Source: CAD feature listing. Evaluate the final solid. Frame: model axes, mm. A direction names the side the tool comes from. Round coordinates to 2 decimals unless told otherwise and drop trailing zeros. Loops run counter-clockwise (first coordinate to the right, second up) from the corner with the lowest first, then second, coordinate; pieces in that order, holes last.
Item 1: Section query B-B on z = 1.4. Return loops of the section in (x, y) (3 decimals), then the cut area to 3 significant figures.
Item 2: Section query D-D on y = 9. Return loops of the section in (x, z), then the cut area to 3 significant figures.
Item 3: Access query for faces 1 (the flat face through (40, 44, 3)), 2 (the flat face through (40, 5, 3)), 3 (the flat face through (-40, 44, 3)). Directions: +Z, -Z, +X, -X, +Y, -Y. A direction counts if a zero-diameter tool reaches every point of the face in a straight line with its end or side. Return the directions, or none.
Item 4: Section query C-C on x = -24. Return loops of the section in (y, z).
Item 5: Ray query, L1, parallel to Y at x = -21, z = 3.25; L2, parallel to X at y = 36, z = 3.6; L3, parallel to Y at x = -25, z = 5.3. Return the intervals inside material, ascending.
Item 6: Pull-direction query (X, two-part tool) for faces 4 (the flat face through (-40, 5, 3)), 5 (the cylindrical face through (22.21, 38.53, 2.96)), 6 (the flat face through (-43, 32, 3)); classes: released by +X, released by -X, zero draft, split by the parting line, or undercut.
Item 7: First-contact query: P1, Ø6.5, axis at x = 22.665, y = 42, coming from the -Z side; P2, Ø3, axis at y = 44, z = 3.5, coming from the -X side; P3, Ø1.8, axis at x = -43, z = 4, coming from the +Y side; P4, Ø1.8, axis at x = -41.5, z = 2, coming from the -Y side. Flat tips, straight axial feed; report the tip coordinate or a pass-through.
Item 8: Section query A-A on y = 42. Return loops of the section in (x, z) (3 decimals).
Autodesk Inventor part; units mm, degrees
ref_plane "YZ Plane" through (0, 0, 0) normal (1, 0, 0) x (0, 1, 0)
ref_plane "XZ Plane" through (0, 0, 0) normal (0, 1, 0) x (-1, 0, 0)
ref_plane "XY Plane" through (0, 0, 0) normal (0, 0, 1) x (1, 0, 0)
sketch "Sketch1" plane through (0, 0, 0) normal (0, 0, 1) x (1, 0, 0)
  line L0 (-40, 0) -> (40, 0)
  circle A0 centre (-22.665, 42) radius 3.5
  circle A1 centre (22.665, 42) radius 3.5
  line L1 (-40, 10) -> (-40, 0)
  line L2 (40, 60) -> (40, 32)
  line L3 (40, 32) -> (46, 32)
  line L4 (46, 32) -> (46, 10)
  line L5 (46, 10) -> (40, 10)
  line L6 (40, 10) -> (40, 0)
  line L7 (-40, 10) -> (-46, 10)
  line L8 (-46, 10) -> (-46, 32)
  line L9 (-46, 32) -> (-40, 32)
  line L10 (-40, 32) -> (-40, 60)
  line L11 (-40, 60) -> (40, 60)
  point P0 (0, 0)
  point P1 (0, 42)
  point P2 (0, 0)
  dimension "d1" = 60
  dimension "d4" = 80
  dimension "d5" = 7
  dimension "d7" = 7
  dimension "d9" = 22.665
  dimension "d10" = 22.665
  dimension "d11" = 42
  dimension "d32" = 6
  dimension "d33" = 28
  dimension "d34" = 10
  dimension "d35" = 10
  dimension "d36" = 28
  dimension "d37" = 6
  dimension "d38" = 6
  dimension "d39" = 22
extrude "Extrusion2" add sketch "Sketch1" along normal blind 6
fillet "Fillet3" radius 4 2 edges at (-40, 60, 3) (40, 60, 3)
equation "\"d1\" = d0"
equation "\"d7\" = d5"
equation "\"d32\" = d28"
equation "\"d33\" = d29"
equation "\"d35\" = d34"
equation "\"d36\" = d33"
equation "\"d37\" = d32"
properties part number "Tope riel final"
Data:
1. outline: (-46, 10) - (-40, 10) - (-40, 0) - (40, 0) - (40, 10) - (46, 10) - (46, 32) - (40, 32) - (40, 56) arc R4 ccw to (36, 60) - (-36, 60) arc R4 ccw to (-40, 56) - (-40, 32) - (-46, 32) - close; hole circle Ø7 at (-22.665, 42); hole circle Ø7 at (22.665, 42)
1. area: 4,980 mm2
2. outline: (-40, 0) - (40, 0) - (40, 6) - (-40, 6) - close
2. area: 480 mm2
3. face 1: +Z, -Z, +X, +Y
3. face 2: +Z, -Z, +X, -Y
3. face 3: +Z, -Z, -X, +Y
4. outline: (0, 0) - (38.76, 0) - (38.76, 6) - (0, 6) - close; (45.24, 0) - (60, 0) - (60, 6) - (45.24, 6) - close
5. L1: y = 0 to 38.92, 45.08 to 60
5. L2: x = -40 to 40
5. L3: y = 0 to 39.39, 44.61 to 60
6. face 4: released by -X
6. face 5: undercut
6. face 6: zero draft
7. P1: passes through
7. P2: stops at x = -40
7. P3: stops at y = 32
7. P4: stops at y = 10
8. outline: (-40, 0) - (-26.165, 0) - (-26.165, 6) - (-40, 6) - close; (-19.165, 0) - (19.165, 0) - (19.165, 6) - (-19.165, 6) - close; (26.165, 0) - (40, 0) - (40, 6) - (26.165, 6) - close
